Geometry check sheet. Reference: the model listing, model coordinates, mm. A direction names the side the tool comes from. Round coordinates to 2 decimals unless told otherwise and drop trailing zeros. Loops run counter-clockwise (first coordinate to the right, second up) from the corner with the lowest first, then second, coordinate; pieces in that order, holes last. Notation, with made-up numbers: M 39,49.25 L 74,49.25 A18 cw 74,66.25 Z; hole C 64,-23.75 d2. An arc over 180 degrees is marked long. Write item = value, one per line.
from build123d import *

# Parameters (mm, degrees)
SKETCH1_W           = 55
SKETCH1_H           = 55
SKETCH1_R           = 1.5
BOSS_EXTRUDE1_DEPTH = 5
SKETCH2_R           = 3.75
SKETCH2_R_2         = 2.51184584
BOSS_EXTRUDE2_DEPTH = 40
SKETCH3_R           = 11.5
CUT_EXTRUDE1_DEPTH  = 15


with BuildPart() as part:
    # Sketch1 → Boss-Extrude1 (new body)
    with BuildSketch(Plane(origin=(0, 0, 0), x_dir=(1, 0, 0), z_dir=(0, 1, 0))):
        Rectangle(SKETCH1_W, SKETCH1_H)
        with Locations(Location((-15.5, 15.5, 0), (0, 0, 270))):
            Circle(SKETCH1_R, mode=Mode.SUBTRACT)
        with Locations(Location((-15.5, -15.5, 0), (0, 0, 90))):
            Circle(SKETCH1_R, mode=Mode.SUBTRACT)
        with Locations(Location((15.5, -15.5, 0), (0, 0, 270))):
            Circle(SKETCH1_R, mode=Mode.SUBTRACT)
        with Locations(Location((15.5, 15.5, 0), (0, 0, 90))):
            Circle(SKETCH1_R, mode=Mode.SUBTRACT)
    extrude(amount=BOSS_EXTRUDE1_DEPTH)

    # Sketch2 → Boss-Extrude2 (add)
    # profile 1 of 4: a face of its own
    with BuildSketch(Plane(origin=(0, 5, 0), x_dir=(1, 0, 0), z_dir=(0, 1, 0))):
        with Locations(Location((-15.77, 0, 0), (0, 0, 90))):
            Circle(SKETCH2_R)
        with Locations(Location((-15.77, 0, 0), (0, 0, 270))):
            Circle(SKETCH2_R_2, mode=Mode.SUBTRACT)
    # profile 2 of 4: a face of its own
    with BuildSketch(Plane(origin=(0, 5, 0), x_dir=(1, 0, 0), z_dir=(0, 1, 0))):
        with Locations(Location((15.77, 0, 0), (0, 0, 90))):
            Circle(SKETCH2_R)
        with Locations(Location((15.77, 0, 0), (0, 0, 90))):
            Circle(SKETCH2_R_2, mode=Mode.SUBTRACT)
    # profile 3 of 4: a face of its own
    with BuildSketch(Plane(origin=(0, 5, 0), x_dir=(1, 0, 0), z_dir=(0, 1, 0))):
        with Locations(Location((0, -15.77, 0), (0, 0, 90))):
            Circle(SKETCH2_R)
        with Locations(Location((0, -15.77, 0), (0, 0, 270))):
            Circle(SKETCH2_R_2, mode=Mode.SUBTRACT)
    # profile 4 of 4: a face of its own
    with BuildSketch(Plane(origin=(0, 5, 0), x_dir=(1, 0, 0), z_dir=(0, 1, 0))):
        with Locations(Location((0, 15.77, 0), (0, 0, 90))):
            Circle(SKETCH2_R)
        with Locations(Location((0, 15.77, 0), (0, 0, 90))):
            Circle(SKETCH2_R_2, mode=Mode.SUBTRACT)
    extrude(amount=BOSS_EXTRUDE2_DEPTH)

    # Sketch3 → Cut-Extrude1 (cut)
    with BuildSketch(Plane(origin=(0, 5, 0), x_dir=(1, 0, 0), z_dir=(0, 1, 0))):
        with Locations(Location((0, 0, 0), (0, 0, 270))):
            Circle(SKETCH3_R)
    extrude(amount=-CUT_EXTRUDE1_DEPTH, mode=Mode.SUBTRACT)


solid = part.part
(1) Material ranges on line 1 along X through (y, z) = (7, 1.5); line 2 along Z through (x, y) = (-15.5, 27); line 3 along X through (y, z) = (7.5, -1), recorded low to high. Write a range as from..to.
Result set:
line_1 = -19.21..-17.78, -13.76..-12.33, 12.33..13.76, 17.78..19.21
line_2 = -3.74..-2.5, 2.5..3.74
line_3 = -19.38..-18.07, -13.47..-12.16, 12.16..13.47, 18.07..19.38
(2) Sectioned sample at A-A on y = 13. Record the cut outline in (x, z), then the cut area to 3 significant figures.
Result set:
outline = C -15.77,0 d7.5; C 0,-15.77 d7.5; C 0,15.77 d7.5; C 15.77,0 d7.5; hole C -15.77,0 d5.02; hole C 0,-15.77 d5.02; hole C 0,15.77 d5.02; hole C 15.77,0 d5.02
area = 97.4 mm2
(3) Tool access check on faces 1 (the cylindrical face through (0.754, 24.72, 18.166)), 2 (the flat face through (-13, 0, 0)). Record the directions out of +Z, -Z, +X, -X, +Y, -Y that give a thin tool (end or side, any length) a straight path to the whole face; none if there is none.
Result set:
face_1 = +Y
face_2 = +Z, -Z, +X, -X, -Y
(4) Depth check by flat-ended pin: pin 1 Ø6 at (x, z) = (0, -15.77) entering from +Y; pin 2 Ø5 at (y, z) = (12, 14) entering from -X; pin 3 Ø1.5 at (x, z) = (15.5, 1) entering from +Y; pin 4 Ø6 at (x, y) = (20, 38.5) entering from -Z. Enter the tip coordinate at first touch or a pass-through.
Result set:
pin_1 = 45
pin_2 = -3.75
pin_3 = 5
pin_4 = -3.54
(5) Sectioned sample at D-D on x = -5. Record the cut outline in (y, z), then the cut area to 3 significant figures.
Result set:
outline = M 0,-27.5 L 5,-27.5 L 5,-10.36 L 0,-10.36 Z; M 0,10.36 L 5,10.36 L 5,27.5 L 0,27.5 Z
area = 171 mm2
(6) Sectioned sample at C-C on y = 4. Record the cut outline in (x, z), then the cut area to 3 significant figures.
Result set:
outline = M -27.5,-27.5 L 27.5,-27.5 L 27.5,27.5 L -27.5,27.5 Z; hole C -15.5,-15.5 d3; hole C -15.5,15.5 d3; hole C 0,0 d23; hole C 15.5,-15.5 d3; hole C 15.5,15.5 d3
area = 2,580 mm2
(7) Sectioned sample at B-B on z = 0. Record the cut outline in (x, y), then the cut area to 3 significant figures.
Result set:
outline = M -27.5,0 L -11.5,0 L -11.5,5 L -12.02,5 L -12.02,45 L -13.26,45 L -13.26,5 L -18.28,5 L -18.28,45 L -19.52,45 L -19.52,5 L -27.5,5 Z; M 11.5,0 L 27.5,0 L 27.5,5 L 19.52,5 L 19.52,45 L 18.28,45 L 18.28,5 L 13.26,5 L 13.26,45 L 12.02,45 L 12.02,5 L 11.5,5 Z
area = 358 mm2
(8) Release check for a two-part mould opening along X. For faces 3 (the cylindrical face through (13.28, 24.72, 0.33)), 4 (the flat face through (-27.5, 2, 0)), 5 (the cylindrical face through (-0.165, 24.72, -12.024)) record: released by +X, released by -X, zero draft, split by the parting line, or undercut.
Result set:
face_3 = undercut
face_4 = released by -X
face_5 = split by the parting line
